Read the model definition and answer for the solid it produces. Units are mm, in the model's axes. A direction names the side the tool comes from. Round coordinates to 2 decimals unless told otherwise and drop trailing zeros. Loops run counter-clockwise (first coordinate to the right, second up) from the corner with the lowest first, then second, coordinate; pieces in that order, holes last. Notation, with made-up numbers: M 80.5,2.5 L 95.5,2.5 A16 cw 95.5,30.5 Z; hole C 65.25,-34 d10. An arc over 180 degrees is marked long. Write each question's results on one line, items separated by ' | '.
```python
from build123d import *

# Parameters (mm, degrees)
SKETCH1_R           = 25
BOSS_EXTRUDE1_DEPTH = 50
SKETCH2_R           = 20
BOSS_EXTRUDE2_DEPTH = 30
SKETCH3_W           = 20
SKETCH3_H           = 10
BOSS_EXTRUDE3_DEPTH = 120
SKETCH4_W           = 20
SKETCH4_H           = 20
BOSS_EXTRUDE4_DEPTH = 50
SKETCH5_W           = 20
SKETCH5_H           = 20
BOSS_EXTRUDE5_DEPTH = 40
SKETCH6_R           = 3
CUT_EXTRUDE1_DEPTH  = 20


with BuildPart() as part:
    # Sketch1 → Boss-Extrude1 (new, symmetric)
    with BuildSketch(Plane(origin=(0, 0, 0), x_dir=(1, 0, 0), z_dir=(0, 1, 0))):
        with Locations(Location((0, 0, 0), (0, 0, 270))):
            Circle(SKETCH1_R)
    extrude(amount=BOSS_EXTRUDE1_DEPTH, both=True)

    # Sketch2 → Boss-Extrude2 (add)
    with BuildSketch(Plane(origin=(0, 0, 0), x_dir=(0, 0, -1), z_dir=(1, 0, 0))):
        with Locations(Location((0, 0, 0), (0, 0, 180))):
            Circle(SKETCH2_R)
    extrude(amount=BOSS_EXTRUDE2_DEPTH)

    # Sketch3 → Boss-Extrude3 (add)
    with BuildSketch(Plane(origin=(0, 0, 0), x_dir=(0, 0, -1), z_dir=(1, 0, 0))):
        with Locations((15, 45)):
            Rectangle(SKETCH3_W, SKETCH3_H)
    extrude(amount=BOSS_EXTRUDE3_DEPTH)

    # Sketch4 → Boss-Extrude4 (add)
    with BuildSketch(Plane.XZ.offset(-40)):
        with Locations((110, -15)):
            Rectangle(SKETCH4_W, SKETCH4_H)
    extrude(amount=BOSS_EXTRUDE4_DEPTH)

    # Sketch5 → Boss-Extrude5 (add)
    with BuildSketch(Plane(origin=(0, 0, -25), x_dir=(-1, 0, 0), z_dir=(0, 0, -1))):
        with Locations((-110, 0)):
            Rectangle(SKETCH5_W, SKETCH5_H)
    extrude(amount=-BOSS_EXTRUDE5_DEPTH)

    # Sketch6 → Cut-Extrude1 (cut)
    with BuildSketch(Plane(origin=(120, 0, 0), x_dir=(0, 0, -1), z_dir=(1, 0, 0))):
        Circle(SKETCH6_R)
    extrude(amount=-CUT_EXTRUDE1_DEPTH, mode=Mode.SUBTRACT)


solid = part.part
```
1. Determine the mould class of faces 1 (the face through (77, 45, -25)), 2 (the face through (110, 0, 15)), 3 (the face through (0, -50, 0)), 4 (the face through (110, 0, 3)) for opening direction Z: released by +Z, released by -Z, zero draft, split by the parting line, or undercut.
Completed:
face 1: released by -Z | face 2: released by +Z | face 3: zero draft | face 4: undercut
2. Which of the six approach directions +Z, -Z, +X, -X, +Y, -Y give full straight-line access (tool end or side, diameter ignored) to faces 5 (the face through (110, -10, -5)), 6 (the face through (24.06, -0.88, -19.98)), 7 (the face through (32, 50, -6)), 8 (the face through (110, 10, 5)), 9 (the face through (30, 0, 0))?
Completed:
face 5: +Z, -Z, +X, -Y | face 6: none | face 7: +Z, -Z, +X, -X, +Y | face 8: +Z, +X, +Y | face 9: +Z, -Z, -Y
3. Find section D-D, the plane x = 84.5. Give the vertices of the cut face in (y, z), then the cut area to 3 significant figures.
Completed:
outline: M 40,-25 L 50,-25 L 50,-5 L 40,-5 Z | area: 200 mm2
4. Find section A-A, the plane z = 0. Give the vertices of the cut face in (x, y).
Completed:
outline: M -25,-50 L 25,-50 L 25,-20 L 30,-20 L 30,20 L 25,20 L 25,50 L -25,50 Z; M 100,-10 L 120,-10 L 120,-3 L 100,-3 Z; M 100,3 L 120,3 L 120,10 L 100,10 Z
5. Find the intervals of material crossed by L1, parallel to Y at x = 104.25, z = 0; L2, parallel to X at y = -9, z = 0.5 (3 decimals); L3, parallel to X at y = 22, z = 15, in increasing order.
Completed:
L1: y = -10 to -3, 3 to 10 | L2: x = -24.995 to 30, 100 to 120 | L3: x = -20 to 20
6. Find section B-B, the plane y = 0. Give the vertices of the cut face in (x, z), then the cut area to 3 significant figures.
Completed:
outline: M 15,-20 L 30,-20 L 30,20 L 15,20 A25 ccw long Z; M 100,-25 L 120,-25 L 120,-3 L 100,-3 Z; M 100,3 L 120,3 L 120,15 L 100,15 Z | area: 2,960 mm2
7. Given P1, Ø2, axis at y = -3.5, z = 18, coming from the +X side; P2, Ø5, axis at y = 26.5, z = 13.5, coming from the -X side; P3, Ø10, axis at x = 93.5, z = 9, coming from the -Y side; P4, Ø22, axis at x = 107.5, y = -1.5, coming from the +Z side, each flat-ended and moving along its own axis, determine where each tip first touches the part or whether it passes through.
Completed:
P1: stops at x = 30 | P2: stops at x = -22.45 | P3: passes through | P4: stops at z = 15
8. Find section C-C, the plane y = 28. Give the vertices of the cut face in (x, z).
Completed:
outline: C 0,0 d50; M 100,-25 L 120,-25 L 120,-5 L 100,-5 Z
